Autodesk Inventor part; units mm, degrees
ref_plane "YZ Plane" through (0, 0, 0) normal (1, 0, 0) x (0, 1, 0)
ref_plane "XZ Plane" through (0, 0, 0) normal (0, 1, 0) x (-1, 0, 0)
ref_plane "XY Plane" through (0, 0, 0) normal (0, 0, 1) x (1, 0, 0)
sketch "Sketch1" plane through (0, 0, 0) normal (0, 1, 0) x (-1, 0, 0)
  point P0 (0, 0)
sketch "Sketch2" plane through (0, 0, 0) normal (0, 1, 0) x (-1, 0, 0)
  line L0 (0, 0) -> (-52.05, 0)
  line L1 (-52.05, 0) -> (-52.05, 88.8)
  line L2 (-52.05, 88.8) -> (0, 88.8)
  line L3 (0, 88.8) -> (0, 0)
  circle A0 centre (-8.975, 47.33) radius 1.9
  line L4 (-26.025, 67.1436) -> (-26.025, 88.8)
  circle A1 centre (-12.075, 4.83) radius 1.6
  circle A2 centre (-43.075, 47.33) radius 1.9
  circle A3 centre (-39.975, 4.83) radius 1.6
  circle A4 centre (-26.025, 20.45) radius 2
  dimension "d0" = 52.05
  dimension "d1" = 88.8
  dimension "d2" = 3.8
  dimension "d4" = 17.05
  dimension "d5" = 3.2
  dimension "d6" = 13.95
  dimension "d7" = 42.5
  dimension "d12" = 4.83
  dimension "d13" = 4
  dimension "d17" = 15.62
  dimension "d18" = 27.9
  dimension "d19" = 3.1
  dimension "d20" = 13.95
extrude "Extrusion1" add sketch "Sketch2" along normal blind 5 contours A0 | A1 | A2 | A3
sketch "Sketch3" plane through (43.075, 0, 47.33) normal (0, -1, 0) x (1, 0, 0)
  circle A0 centre (0, 0) radius 1.9
  circle A1 centre (-34.1, 0) radius 1.9
  point P0 (-43.075, -47.33)
  dimension "d21" = 34.1
extrude "Extrusion2" add sketch "Sketch2" along normal blind 1 contours L0 L1 L2 L3 | A4
extrude "Extrusion3" cut sketch "Sketch2" along normal mid plane 5 contours A4
properties part number "test fit for rfid reader"
Work out the finished part from the listing and answer in its coordinate system (mm). A direction names the side the tool comes from. Give positions to 0.01 mm unless a question says otherwise; leave off trailing zeros. Order: outer loops, then holes, each group sorted by start corner. A loop starts at its lowest first (then second) coordinate and runs counter-clockwise, first axis right, second up. Notation, with made-up numbers: (15, -39.75) -> (44, -39.75) arc R20 cw to (44, -34.75) -> close; hole circle Ø7 at (-17.5, -12). An arc over 180 degrees is marked (long way). One line per item, written item: value.
Item 1: Flat-ended cylindrical pins translate along their axes: P1, Ø5, axis at x = 26.025, z = 20.45, coming from the +Y side; P2, Ø1.5, axis at x = 30, z = 79.5, coming from the -Y side. Find the tip coordinate at first contact, or state that the pin passes through.
Answer sheet:
P1: y = 1
P2: y = 0
Item 2: Determine the mould class of faces 1 (the cylindrical face through (40.322, 2.972, 6.392)), 2 (the flat face through (12, 5, 5)) for opening direction X: released by +X, released by -X, zero draft, split by the parting line, or undercut.
Answer sheet:
face 1: undercut
face 2: zero draft
Item 3: Find section D-D, the plane y = 3.55. Give the vertices of the cut face in (x, z) (3 decimals), plus the area to 3 significant figures.
Answer sheet:
outline: circle Ø3.8 at (8.975, 47.33); circle Ø3.2 at (12.075, 4.83); circle Ø3.2 at (39.975, 4.83); circle Ø3.8 at (43.075, 47.33)
area: 38.8 mm²
Item 4: Find section C-C, the plane x = 4.5. Give the vertices of the cut face in (y, z), plus the area to 3 significant figures.
Answer sheet:
outline: (0, 0) -> (1, 0) -> (1, 88.8) -> (0, 88.8) -> close
area: 88.8 mm²
Item 5: Straight lines are drawn through the part: probe 1 along X at (y, z) = (0.65, 20.45) (3 decimals); probe 2 along Y at (x, z) = (16, 69); probe 3 along X at (y, z) = (3.4, 46). For each, find the intervals that lie inside material, in ascending order.
Answer sheet:
probe 1: 0 to 24.025, 28.025 to 52.05
probe 2: 0 to 1
probe 3: 7.62 to 10.33, 41.72 to 44.43
Item 6: Find section B-B, the plane z = 47.33. Give the vertices of the cut face in (x, y) (3 decimals).
Answer sheet:
outline: (0, 0) -> (52.05, 0) -> (52.05, 1) -> (44.975, 1) -> (44.975, 5) -> (41.175, 5) -> (41.175, 1) -> (10.875, 1) -> (10.875, 5) -> (7.075, 5) -> (7.075, 1) -> (0, 1) -> close
Item 7: A tool of negligible diameter and unlimited length cuts with its end or side. For faces 3 (the cylindrical face through (11.34, 2.97, 6.25)), 4 (the flat face through (43, 5, 47)), from which of +Z, -Z, +X, -X, +Y, -Y can it reach the whole face along a straight path? Write none if from no direction.
Answer sheet:
face 3: +Y
face 4: +Z, -Z, +X, -X, +Y
Item 8: Find section A-A, the plane z = 20.45. Give the vertices of the cut face in (x, y) (3 decimals), plus the area to 4 significant figures.
Answer sheet:
outline: (0, 0) -> (24.025, 0) -> (24.025, 1) -> (0, 1) -> close; (28.025, 0) -> (52.05, 0) -> (52.05, 1) -> (28.025, 1) -> close
area: 48.05 mm²
